Verification items for the finished model (mm, model axes). Coordinates: 2 decimals unless noted, no trailing zeros. Loops run counter-clockwise (first coordinate to the right, second up) from the corner with the lowest first, then second, coordinate; pieces in that order, holes last. Notation, with made-up numbers: M 26.5,-5 L 40.5,-5 A28 cw 40.5,18 Z; hole C 39.25,16 d7. An arc over 180 degrees is marked long. Write item = value, one per line. Start each with the question number.
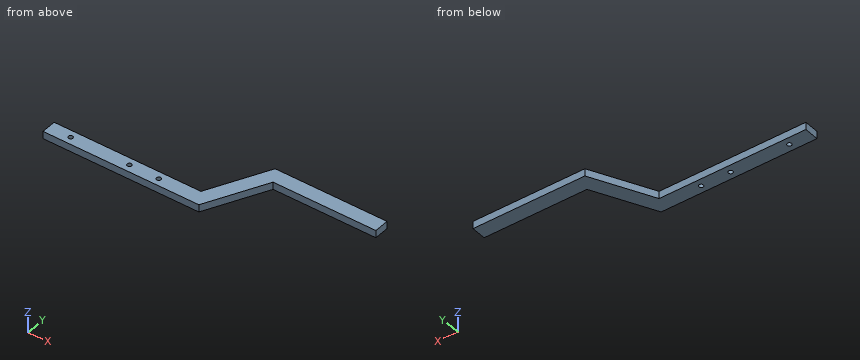
```python
from build123d import *

# Parameters (mm, degrees)
F0_R     = 1.5
F1_DEPTH = 5
F2_DEPTH = 265


# Not quite as in the source:
# - an extrude ends at something that could not be found from the text; its depth is read off the source's solid


with BuildPart() as f1:
    # F0 (on Top) → F1 (new body)
    with BuildSketch(Plane.XY):
        Polygon((-52.0408339798, -45.9276453106), (-151.9144345724, -45.9276453106), (-151.9144345724, -55.9276454151), (-45.8887560524, -55.9276454151), (-25.683571109, -15.9276453106), (27.9570557177, -15.9276453106), (44.264588505, -15.9276453106), (44.264588505, -5.9276453106), (27.9570557177, -5.9276453106), (-31.8356490892, -5.9276453106), (-31.9144345724, -6.0836161342), align=None)
        with Locations((-136.9144345724, -50.9276454151)):
            Circle(F0_R, mode=Mode.SUBTRACT)
        with Locations((-96.9144345724, -50.9276454151)):
            Circle(F0_R, mode=Mode.SUBTRACT)
        with Locations((-76.9144345724, -50.9276454151)):
            Circle(F0_R, mode=Mode.SUBTRACT)
    extrude(amount=F1_DEPTH)

    # F0 (on Top) → F2 (cut, through all)
    with BuildSketch(Plane.XY):
        with Locations((-76.9144345724, -50.9276454151)):
            Circle(F0_R)
        with Locations((-96.9144345724, -50.9276454151)):
            Circle(F0_R)
    extrude(amount=-F2_DEPTH, mode=Mode.SUBTRACT)


solid = f1.part
```
Q1. Sectioned sample at B-B on x = 28. Record the cut outline in (y, z), plus the area to 3 significant figures.
Q2. Sectioned sample at A-A on z = 3.15. Record the cut outline in (x, y).
Q3. Scan lines: L1, parallel to X at y = -50.5, z = 4.55; L2, parallel to Y at x = -78.5, z = 2.9; L3, parallel to Y at x = 3.5, z = 1.2. Record each from-to range of solid material in increasing order. Write a range as [from, to].
Q4. Sectioned sample at C-C on y = -10. Record the cut outline in (x, z), plus the area to 3 significant figures.
Q5. Gauge pin test, flat ends, axial feed: pin 1 (1 mm diameter, centred on x = -126, z = 1, fed in from +Y); pin 2 (2 mm diameter, centred on y = -30.5, z = 3, fed in from -X); pin 3 (2 mm diameter, centred on y = -28, z = 4.5, fed in from -X); pin 4 (2.5 mm diameter, centred on x = -136.91, y = -50.93, fed in from -Z). Record the tip position at first contact, or that the pin passes through.
Solutions:
q1.outline = M -15.93,0 L -5.93,0 L -5.93,5 L -15.93,5 Z
q1.area = 50.0 mm²
q2.outline = M -151.91,-55.93 L -45.89,-55.93 L -25.68,-15.93 L 44.26,-15.93 L 44.26,-5.93 L -31.84,-5.93 L -52.04,-45.93 L -151.91,-45.93 Z; hole C -136.91,-50.93 d3; hole C -96.91,-50.93 d3; hole C -76.91,-50.93 d3
q3.L1 = [-151.91, -138.35], [-135.48, -98.35], [-95.48, -78.35], [-75.48, -43.15]
q3.L2 = [-55.93, -45.93]
q3.L3 = [-15.93, -5.93]
q4.outline = M -33.89,0 L 44.26,0 L 44.26,5 L -33.89,5 Z
q4.area = 391 mm²
q5.pin_1 = -45.93
q5.pin_2 = -44.75
q5.pin_3 = -43.49
q5.pin_4 = through
